Input: part model. Units: mm. Frame: model coordinates. Give positions to 0.01 mm unless a question says otherwise; leave off trailing zeros. Order: outer loops, then holes, each group sorted by start corner. A loop starts at its lowest first (then second) coordinate and runs counter-clockwise, first axis right, second up. Notation, with made-up numbers: (60.25, -33.5) - (103.25, -33.5) arc R22 cw to (103.25, -1.5) - close; hole circle Ø7 at (44, 51). An arc over 180 degrees is marked (long way). Answer in a Markdown table with one row per item. Add a question column.
from build123d import *

# Parameters (mm, degrees)
F0_R     = 359.41
F0_R_2   = 9.525
F0_R_3   = 320.294
F1_DEPTH = 12.7


with BuildPart() as f1:
    # F0 (on Front) → F1 (new body)
    with BuildSketch(Plane.XZ):
        Circle(F0_R)
        with Locations((-190.505033, -285.11093)):
            Circle(F0_R_2, mode=Mode.SUBTRACT)
        with Locations((-285.11093, -190.505033)):
            Circle(F0_R_2, mode=Mode.SUBTRACT)
        with Locations((-242.466915, -242.466915)):
            Circle(F0_R_2, mode=Mode.SUBTRACT)
        with Locations((-131.222149, -316.798292)):
            Circle(F0_R_2, mode=Mode.SUBTRACT)
        with Locations((-66.896471, -336.311273)):
            Circle(F0_R_2, mode=Mode.SUBTRACT)
        with Locations((-316.798292, -131.222149)):
            Circle(F0_R_2, mode=Mode.SUBTRACT)
        with Locations((-336.311273, -66.896471)):
            Circle(F0_R_2, mode=Mode.SUBTRACT)
        with Locations((0, -342.9)):
            Circle(F0_R_2, mode=Mode.SUBTRACT)
        with Locations((66.896471, -336.311273)):
            Circle(F0_R_2, mode=Mode.SUBTRACT)
        with Locations((131.222149, -316.798292)):
            Circle(F0_R_2, mode=Mode.SUBTRACT)
        with Locations((190.505033, -285.11093)):
            Circle(F0_R_2, mode=Mode.SUBTRACT)
        with Locations((242.466915, -242.466915)):
            Circle(F0_R_2, mode=Mode.SUBTRACT)
        with Locations((285.11093, -190.505033)):
            Circle(F0_R_2, mode=Mode.SUBTRACT)
        with Locations((316.798292, -131.222149)):
            Circle(F0_R_2, mode=Mode.SUBTRACT)
        with Locations((336.311273, -66.896471)):
            Circle(F0_R_2, mode=Mode.SUBTRACT)
        with Locations((-342.9, 0)):
            Circle(F0_R_2, mode=Mode.SUBTRACT)
        with Locations((-336.311273, 66.896471)):
            Circle(F0_R_2, mode=Mode.SUBTRACT)
        with Locations((-316.798292, 131.222149)):
            Circle(F0_R_2, mode=Mode.SUBTRACT)
        with Locations((-285.11093, 190.505033)):
            Circle(F0_R_2, mode=Mode.SUBTRACT)
        with Locations((-242.466915, 242.466915)):
            Circle(F0_R_2, mode=Mode.SUBTRACT)
        with Locations((-190.505033, 285.11093)):
            Circle(F0_R_2, mode=Mode.SUBTRACT)
        with Locations((-131.222149, 316.798292)):
            Circle(F0_R_2, mode=Mode.SUBTRACT)
        with Locations((-66.896471, 336.311273)):
            Circle(F0_R_2, mode=Mode.SUBTRACT)
        Circle(F0_R_3, mode=Mode.SUBTRACT)
        with Locations((342.9, 0)):
            Circle(F0_R_2, mode=Mode.SUBTRACT)
        with Locations((336.311273, 66.896471)):
            Circle(F0_R_2, mode=Mode.SUBTRACT)
        with Locations((316.798292, 131.222149)):
            Circle(F0_R_2, mode=Mode.SUBTRACT)
        with Locations((0, 342.9)):
            Circle(F0_R_2, mode=Mode.SUBTRACT)
        with Locations((66.896471, 336.311273)):
            Circle(F0_R_2, mode=Mode.SUBTRACT)
        with Locations((131.222149, 316.798292)):
            Circle(F0_R_2, mode=Mode.SUBTRACT)
        with Locations((242.466915, 242.466915)):
            Circle(F0_R_2, mode=Mode.SUBTRACT)
        with Locations((285.11093, 190.505033)):
            Circle(F0_R_2, mode=Mode.SUBTRACT)
        with Locations((190.505033, 285.11093)):
            Circle(F0_R_2, mode=Mode.SUBTRACT)
    extrude(amount=F1_DEPTH)


solid = f1.part
Q1. Pull-direction query (X, two-part tool) for faces 1 (the flat face through (-321, -12.7, 2)), 2 (the cylindrical face through (-77.913, -6.261, -350.863)), 3 (the cylindrical face through (305.503, -6.261, 96.208)); classes: +X half, -X half, draft (parallel to the pull), parting line (faces both ways), or undercut.
Q2. Section B-B, the plane z = 0. Return loops of the section in (x, y) (3 decimals).
Q3. Section D-D, the plane y = -4.5. State how many separate pieces and enclosed holes the cut face has, then the cut area to 3 significant figures.
Q4. Line query: probe 1 along Z at (x, y) = (-195, -7.25); probe 2 along Z at (x, y) = (-237, -9); probe 3 along Z at (x, y) = (-26.5, -1.75). Output: solid intervals per line, ascending.
Q5. Contact query for flat-ended pins moving along their axis: P1, Ø3, axis at y = -7, z = 272.5, coming from the -X side; P2, Ø22, axis at x = 336.31, z = -66.9, coming from the +Y side; P3, Ø15, axis at x = 342.9, z = 0, coming from the +Y side; P4, Ø6, axis at x = -273.5, y = -4, coming from the -Z side. Output: stop coordinate, or through.
Q6. Section C-C, the plane z = -158. Return loops of the section in (x, y), then the cut area to 3 significant figures.
Q7. Section A-A, the plane x = 0. Return loops of the section in (y, z) (3 decimals), then the cut area to 3 significant figures.
Computed:
| question | item | result |
|---|---|---|
| 1 | face 1 | draft |
| 1 | face 2 | parting line |
| 1 | face 3 | undercut |
| 2 | outline | (-359.41, -12.7) - (-352.425, -12.7) - (-352.425, 0) - (-359.41, 0) - close; (-333.375, -12.7) - (-320.294, -12.7) - (-320.294, 0) - (-333.375, 0) - close; (320.294, -12.7) - (333.375, -12.7) - (333.375, 0) - (320.294, 0) - close; (352.425, -12.7) - (359.41, -12.7) - (359.41, 0) - (352.425, 0) - close |
| 3 | separate pieces | 1 |
| 3 | enclosed holes | 33 |
| 3 | area | 74,400 mm^2 |
| 4 | probe 1 | z = -301.91 to -293.51, -276.71 to -254.09, 254.09 to 276.71, 293.51 to 301.91 |
| 4 | probe 2 | z = -270.2 to -250.27, -234.67 to -215.45, 215.45 to 234.67, 250.27 to 270.2 |
| 4 | probe 3 | z = -358.43 to -319.2, 319.2 to 358.43 |
| 5 | P1 | stops at x = -236.08 |
| 5 | P2 | stops at y = 0 |
| 5 | P3 | passes through |
| 5 | P4 | stops at z = -236.65 |
| 6 | outline | (-322.82, -12.7) - (-278.61, -12.7) - (-278.61, 0) - (-322.82, 0) - close; (278.61, -12.7) - (322.82, -12.7) - (322.82, 0) - (278.61, 0) - close |
| 6 | area | 1,120 mm^2 |
| 7 | outline | (-12.7, -359.41) - (0, -359.41) - (0, -352.425) - (-12.7, -352.425) - close; (-12.7, -333.375) - (0, -333.375) - (0, -320.294) - (-12.7, -320.294) - close; (-12.7, 320.294) - (0, 320.294) - (0, 333.375) - (-12.7, 333.375) - close; (-12.7, 352.425) - (0, 352.425) - (0, 359.41) - (-12.7, 359.41) - close |
| 7 | area | 510 mm^2 |
